Build history of the part. All positions in model axes, mm. A direction names the side the tool comes from. Round coordinates to 2 decimals unless told otherwise and drop trailing zeros. Loops run counter-clockwise (first coordinate to the right, second up) from the corner with the lowest first, then second, coordinate; pieces in that order, holes last. Notation, with made-up numbers: (65, 71.5) -> (93, 71.5) arc R13 ccw to (93, 96.5) -> close; hole circle Ø7 at (74.5, 89.5). An arc over 180 degrees is marked (long way). Put each result on its own line as item: value. Start each with the question number.
Item 1: Flat gauge pins, fed straight in: pin 1 Ø1.5 at (y, z) = (-5, -2.5) entering from +X; pin 2 Ø4 at (y, z) = (-10.5, 0) entering from +X; pin 3 Ø2 at (y, z) = (-10, 2) entering from -X. Where does each tip first touch, or does it go through?
Item 2: Tool access for faces 4 (the flat face through (1, -1, -3.5)), 5 (the flat face through (0, -2.8, 2.2)): list every direction of +Z, -Z, +X, -X, +Y, -Y with a clear straight run to the whole face (end or side of a thin tool).
Item 3: Cut at A-A, the plane x = 0. List the corners of the cut face in (y, z).
Item 4: Cut at B-B, the plane y = -2. List the corners of the cut face in (x, z).
Item 5: Pull direction X, two halves, no side cores. Call faces 1 (the flat face through (0, -12.8, 0)), 2 (the cylindrical face through (-0.098, -0.656, 0.049)), 3 (the cylindrical face through (2, -7, 0)): +X half, -X half, draft (parallel to the pull), parting line (faces both ways), or undercut.
Item 6: Drill centre lines: probe 1 along Y at (x, z) = (0, 1); probe 2 along Y at (x, z) = (2.25, 0); probe 3 along Z at (x, y) = (-3, -1.5). Where is each one in solid material? Low to high. Write a range as [from, to].
```python
from build123d import *

# Parameters (mm, degrees)
EXTRUDE_1_DEPTH     = 2.8
SKETCH_5_R          = 2
EXTRUDE_2_DEPTH     = 10
CHAMFER_1_SIZE      = 0.5
SKETCH_6_R          = 0.75
CUT_EXTRUDE_1_DEPTH = 16.138471962


with BuildPart() as part:
    # Эскиз1 → Вытянуть1 (new body)
    with BuildSketch(Plane(origin=(0, 0, 0), x_dir=(1, 0, 0), z_dir=(0, 1, 0))):
        Polygon((-2.020725942, 3.5), (2.020725942, 3.5), (4.041451884, 0), (2.020725942, -3.5), (-2.020725942, -3.5), (-4.041451884, 0), align=None)
    extrude(amount=-EXTRUDE_1_DEPTH)

    # Эскиз5 → Вытянуть2 (add)
    with BuildSketch(Plane.XZ.offset(2.8)):
        with Locations(Location((0, 0, 0), (0, 0, 90))):
            Circle(SKETCH_5_R)
    extrude(amount=EXTRUDE_2_DEPTH)

    # Фаска1
    chamfer_1_edges = [part.edges().sort_by_distance(p)[0] for p in [
        (0, -12.8, -2),
    ]]
    chamfer(chamfer_1_edges, length=CHAMFER_1_SIZE)

    # Эскиз4 → Вырез-Повернуть1 (revolve, cut)
    with BuildSketch(Plane.XY, mode=Mode.PRIVATE) as cut_revolve_1_sk:
        Polygon((-4.041451884, -0.6), (-3.441451884, 0), (-4.041451884, 0), align=None)
        Polygon((-4.041451884, -2.2), (-3.441451884, -2.8), (-4.041451884, -2.8), align=None)
    revolve(cut_revolve_1_sk.sketch.rotate(Axis((0, -2.8, 0), (0, -1, 0)), 120.000000136), axis=Axis((0, -2.8, 0), (0, -1, 0)), mode=Mode.SUBTRACT)

    # Эскиз6 → Вырез-Вытянуть1 (cut, through all)
    with BuildSketch(Plane.XY.offset(3.5)):
        with Locations((0, -1.4)):
            Circle(SKETCH_6_R)
    extrude(amount=-CUT_EXTRUDE_1_DEPTH, mode=Mode.SUBTRACT)


solid = part.part
```
Reply:
1. pin 1: stops at x = 0.97
1. pin 2: stops at x = 2
1. pin 3: stops at x = -1.73
2. face 4: -Z, +X, -X, +Y, -Y
2. face 5: -Y
3. outline: (-12.8, -1.5) -> (-12.3, -2) -> (-2.8, -2) -> (-2.8, -3.44) -> (-2.74, -3.5) -> (-2.15, -3.5) -> (-2.15, 3.5) -> (-2.74, 3.5) -> (-2.8, 3.44) -> (-2.8, 2) -> (-12.3, 2) -> (-12.8, 1.5) -> close; (-0.65, -3.5) -> (-0.06, -3.5) -> (0, -3.44) -> (0, 3.44) -> (-0.06, 3.5) -> (-0.65, 3.5) -> close
4. outline: (-4.04, 0) -> (-2.02, -3.5) -> (-0.45, -3.5) -> (-0.45, 3.5) -> (-2.02, 3.5) -> close; (0.45, -3.5) -> (2.02, -3.5) -> (4.04, 0) -> (2.02, 3.5) -> (0.45, 3.5) -> close
5. face 1: draft
5. face 2: undercut
5. face 3: parting line
6. probe 1: y = [-12.8, -2.15], [-0.65, 0]
6. probe 2: y = [-2.8, 0]
6. probe 3: z = [-1.8, 1.8]
